For this review, take the finished solid that the model builds, in its own axes (mm). Face numbers are marked on the shaded views. A direction names the side the tool comes from. Give positions to 0.01 mm unless a question says otherwise; leave off trailing zeros. Loops run counter-clockwise (first coordinate to the right, second up) from the corner with the lowest first, then second, coordinate; pieces in that order, holes last. Notation, with made-up numbers: (-33.75, 73) - (-18.75, 73) arc R13 cw to (-18.75, 92) - close; hole circle Ø10 at (4.25, 43). An arc over 180 degrees is marked (long way). Put each result on its own line as item: value. Start each with the question number.
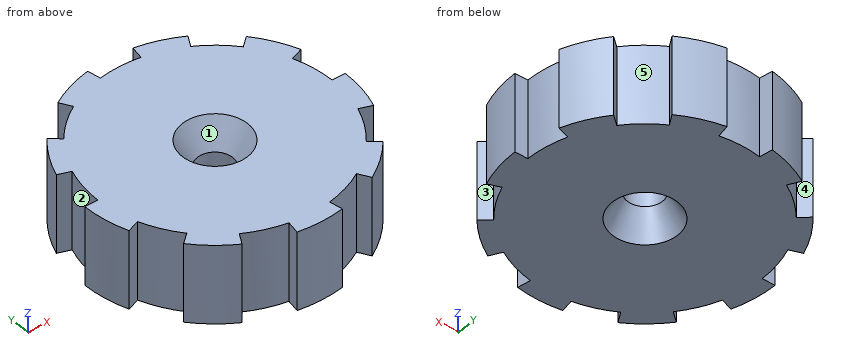
from build123d import *

# Parameters (mm, degrees)
BOSS_EXTRUDE1_DEPTH = 30
SKETCH_2_R          = 12.5
CUT_EXTRUDE1_DEPTH  = 10
CUT_EXTRUDE1_TAPER  = 30
SKETCH3_OUTSIDE_W   = 142.356
SKETCH3_OUTSIDE_H   = 141.596
SKETCH3_OUTSIDE_R   = 12.5
CUT_EXTRUDE4_DEPTH  = 10
CUT_EXTRUDE4_TAPER  = 30
SKETCH8_R           = 6.726497308
CUT_EXTRUDE5_DEPTH  = 60


with BuildPart() as part:
    # Sketch1 → Boss-Extrude1 (new body)
    with BuildSketch(Plane.XY):
        with BuildLine():
            Line((-7.814167995, 44.316348886), (-8.682408883, 49.240387651))
            ThreePointArc((-8.682408883, 49.240387651), (-17.101007166, 46.984631039), (-25, 43.301270189))
            Line((-25, 43.301270189), (-22.5, 38.97114317))
            ThreePointArc((-22.5, 38.97114317), (-28.925442436, 34.47199994), (-34.47199994, 28.925442436))
            Line((-34.47199994, 28.925442436), (-38.302222156, 32.139380484))
            ThreePointArc((-38.302222156, 32.139380484), (-43.301270189, 25), (-46.984631039, 17.101007166))
            Line((-46.984631039, 17.101007166), (-42.286167935, 15.39090645))
            ThreePointArc((-42.286167935, 15.39090645), (-44.316348886, 7.814167995), (-45, 0))
            Line((-45, 0), (-50, 0))
            ThreePointArc((-50, 0), (-49.240387651, -8.682408883), (-46.984631039, -17.101007166))
            Line((-46.984631039, -17.101007166), (-42.286167935, -15.39090645))
            ThreePointArc((-42.286167935, -15.39090645), (-38.97114317, -22.5), (-34.47199994, -28.925442436))
            Line((-34.47199994, -28.925442436), (-38.302222156, -32.139380484))
            ThreePointArc((-38.302222156, -32.139380484), (-32.139380484, -38.302222156), (-25, -43.301270189))
            Line((-25, -43.301270189), (-22.5, -38.97114317))
            ThreePointArc((-22.5, -38.97114317), (-15.39090645, -42.286167935), (-7.814167995, -44.316348886))
            Line((-7.814167995, -44.316348886), (-8.682408883, -49.240387651))
            ThreePointArc((-8.682408883, -49.240387651), (0, -50), (8.682408883, -49.240387651))
            Line((8.682408883, -49.240387651), (7.814167995, -44.316348886))
            ThreePointArc((7.814167995, -44.316348886), (15.39090645, -42.286167935), (22.5, -38.97114317))
            Line((22.5, -38.97114317), (25, -43.301270189))
            ThreePointArc((25, -43.301270189), (32.139380484, -38.302222156), (38.302222156, -32.139380484))
            Line((38.302222156, -32.139380484), (34.47199994, -28.925442436))
            ThreePointArc((34.47199994, -28.925442436), (38.97114317, -22.5), (42.286167935, -15.39090645))
            Line((42.286167935, -15.39090645), (46.984631039, -17.101007166))
            ThreePointArc((46.984631039, -17.101007166), (49.240387651, -8.682408883), (50, 0))
            Line((50, 0), (45, 0))
            ThreePointArc((45, 0), (44.316348886, 7.814167995), (42.286167935, 15.39090645))
            Line((42.286167935, 15.39090645), (46.984631039, 17.101007166))
            ThreePointArc((46.984631039, 17.101007166), (43.301270189, 25), (38.302222156, 32.139380484))
            Line((38.302222156, 32.139380484), (34.47199994, 28.925442436))
            ThreePointArc((34.47199994, 28.925442436), (28.925442436, 34.47199994), (22.5, 38.97114317))
            Line((22.5, 38.97114317), (25, 43.301270189))
            ThreePointArc((25, 43.301270189), (17.101007166, 46.984631039), (8.682408883, 49.240387651))
            Line((8.682408883, 49.240387651), (7.814167995, 44.316348886))
            ThreePointArc((7.814167995, 44.316348886), (0, 45), (-7.814167995, 44.316348886))
        make_face()
    extrude(amount=BOSS_EXTRUDE1_DEPTH)

    # Sketch 2 → Cut-Extrude1 (cut)
    with BuildSketch(Plane.XY.offset(30)):
        Circle(SKETCH_2_R)
    extrude(amount=-CUT_EXTRUDE1_DEPTH, taper=CUT_EXTRUDE1_TAPER, mode=Mode.SUBTRACT)

    # Sketch3 outside → Cut-Extrude4 (cut)
    with BuildSketch(Plane(origin=(0, 0, 0), x_dir=(-1, 0, 0), z_dir=(0, 0, -1))):
        with Locations((0, -0.38)):
            Rectangle(SKETCH3_OUTSIDE_W, SKETCH3_OUTSIDE_H)
        with BuildLine():
            Line((-7.814167995, 44.316348886), (-8.682408883, 49.240387651))
            ThreePointArc((-8.682408883, 49.240387651), (-17.101007166, 46.984631039), (-25, 43.301270189))
            Line((-25, 43.301270189), (-22.5, 38.97114317))
            ThreePointArc((-22.5, 38.97114317), (-28.925442436, 34.47199994), (-34.47199994, 28.925442436))
            Line((-34.47199994, 28.925442436), (-38.302222156, 32.139380484))
            ThreePointArc((-38.302222156, 32.139380484), (-43.301270189, 25), (-46.984631039, 17.101007166))
            Line((-46.984631039, 17.101007166), (-42.286167935, 15.39090645))
            ThreePointArc((-42.286167935, 15.39090645), (-44.316348886, 7.814167995), (-45, 0))
            Line((-45, 0), (-50, 0))
            ThreePointArc((-50, 0), (-49.240387651, -8.682408883), (-46.984631039, -17.101007166))
            Line((-46.984631039, -17.101007166), (-42.286167935, -15.39090645))
            ThreePointArc((-42.286167935, -15.39090645), (-38.97114317, -22.5), (-34.47199994, -28.925442436))
            Line((-34.47199994, -28.925442436), (-38.302222156, -32.139380484))
            ThreePointArc((-38.302222156, -32.139380484), (-32.139380484, -38.302222156), (-25, -43.301270189))
            Line((-25, -43.301270189), (-22.5, -38.97114317))
            ThreePointArc((-22.5, -38.97114317), (-15.39090645, -42.286167935), (-7.814167995, -44.316348886))
            Line((-7.814167995, -44.316348886), (-8.682408883, -49.240387651))
            ThreePointArc((-8.682408883, -49.240387651), (0, -50), (8.682408883, -49.240387651))
            Line((8.682408883, -49.240387651), (7.814167995, -44.316348886))
            ThreePointArc((7.814167995, -44.316348886), (15.39090645, -42.286167935), (22.5, -38.97114317))
            Line((22.5, -38.97114317), (25, -43.301270189))
            ThreePointArc((25, -43.301270189), (32.139380484, -38.302222156), (38.302222156, -32.139380484))
            Line((38.302222156, -32.139380484), (34.47199994, -28.925442436))
            ThreePointArc((34.47199994, -28.925442436), (38.97114317, -22.5), (42.286167935, -15.39090645))
            Line((42.286167935, -15.39090645), (46.984631039, -17.101007166))
            ThreePointArc((46.984631039, -17.101007166), (49.240387651, -8.682408883), (50, 0))
            Line((50, 0), (45, 0))
            ThreePointArc((45, 0), (44.316348886, 7.814167995), (42.286167935, 15.39090645))
            Line((42.286167935, 15.39090645), (46.984631039, 17.101007166))
            ThreePointArc((46.984631039, 17.101007166), (43.301270189, 25), (38.302222156, 32.139380484))
            Line((38.302222156, 32.139380484), (34.47199994, 28.925442436))
            ThreePointArc((34.47199994, 28.925442436), (28.925442436, 34.47199994), (22.5, 38.97114317))
            Line((22.5, 38.97114317), (25, 43.301270189))
            ThreePointArc((25, 43.301270189), (17.101007166, 46.984631039), (8.682408883, 49.240387651))
            Line((8.682408883, 49.240387651), (7.814167995, 44.316348886))
            ThreePointArc((7.814167995, 44.316348886), (0, 45), (-7.814167995, 44.316348886))
        make_face(mode=Mode.SUBTRACT)
        Circle(SKETCH3_OUTSIDE_R)
    extrude(amount=-CUT_EXTRUDE4_DEPTH, taper=CUT_EXTRUDE4_TAPER, mode=Mode.SUBTRACT)

    # Sketch8 → Cut-Extrude5 (cut)
    with BuildSketch(Plane.XY.offset(20)):
        Circle(SKETCH8_R)
    extrude(amount=-CUT_EXTRUDE5_DEPTH, mode=Mode.SUBTRACT)


solid = part.part
1) Insertion check: P1, Ø6, axis at x = 11.5, y = -0.5, coming from the +Z side; P2, Ø4, axis at x = 14.5, z = 7, coming from the -Y side; P3, Ø12, axis at x = 0, y = 0, coming from the -Z side; P4, Ø2, axis at y = 36, z = 4.5, coming from the +X side. Each pin has a flat end and moves straight along its axis. Give the tip position at first contact, or say it passes through.
2) Take a section at A-A on x = 0. State the section outline as (y, z) points.
3) Take a section at C-C on x = 31.5. State the section outline as (y, z) points.
4) Wall thickness on probe 1 along Y at (x, z) = (-36.5, 16.5); probe 2 along Y at (x, z) = (-38, 18.5); probe 3 along X at (y, z) = (18.5, 13): over which ranges is each line inside the solid? List them lowest first.
5) Machinability: for the marked faces 1, 2, 3, 4 and 5, which of the approach directions +Z, -Z, +X, -X, +Y, -Y give a long, thin tool a straight path to every point of the face, cutting with its end or side? Answer none if there is none.
6) Take a section at B-B on y = 23. State the section outline as (x, z) points.
Answers follow:
1. P1: z = 30
1. P2: y = -43.23
1. P3: through
1. P4: x = 28.28
2. outline: (-50, 0) - (-12.5, 0) - (-6.73, 10) - (-6.73, 20) - (-12.5, 30) - (-50, 30) - close; (6.73, 10) - (12.5, 0) - (45, 0) - (45, 30) - (12.5, 30) - (6.73, 20) - close
3. outline: (-38.83, 0) - (32.14, 0) - (32.14, 30) - (-38.83, 30) - close
4. probe 1: -34.17 to -30.63, -26.32 to 30.63
4. probe 2: -32.5 to -31.89, -24.1 to 31.89
4. probe 3: -46.45 to 46.45
5. face 1: +Z
5. face 2: +Z, -Z, -X
5. face 3: +Z, -Z, +X
5. face 4: +Z, -Z, +Y
5. face 5: +Z, -Z
6. outline: (-44.4, 0) - (44.4, 0) - (44.4, 30) - (-44.4, 30) - close
